Could you check a few things on this model? Use its own coordinates, in mm. Face numbers are marked on the shaded views. A direction names the side the tool comes from. Give positions to 0.01 mm unless a question says otherwise; leave off trailing zeros. Loops run counter-clockwise (first coordinate to the right, second up) from the corner with the lowest first, then second, coordinate; pieces in that order, holes last.
1. Imagine slicing it at C-C (x = 15). List the corners of the cut face in (y, z) for me, plus the area to 3 significant figures.
2. For P1, Ø6.5, axis at x = 19.5, y = 15, coming from the +Z side; P2, Ø10, axis at x = 22, z = 13.5, coming from the -Y side; P3, Ø7.5, axis at y = 8.5, z = 13.5, coming from the +X side; P4, Ø10, axis at x = 18, y = 4.5, coming from the -Z side, each with a flat end and sliding along its axis, tell me the tip position at first contact or that it passes through.
3. For the marked faces 1, 2 and 3, which set-ups out of +Z, -Z, +X, -X, +Y, -Y let a thin tool reach every point of the face, with its end or its side?
4. Thinking about a two-plate mould opening in X: for the marked faces 4, 5 and 6, which applies, +X half, -X half, draft (parallel to the pull), parting line (faces both ways), or undercut?
5. Imagine slicing it at B-B (y = 21). List the corners of the cut face in (x, z) for me (3 decimals).
6. Imagine slicing it at A-A (z = 8). List the corners of the cut face in (x, y) for me.
7. I need wall thicknesses on line 1 along X through (y, z) = (22.75, 5.75) (3 decimals); line 2 along Z through (x, y) = (25.4, 14.5) (3 decimals); line 3 along X through (y, z) = (23.75, 14.75). Which ranges of each line are inside material? Lowest first, please.
8. Imagine slicing it at D-D (z = 21.25). List the corners of the cut face in (x, y) for me.
```python
from build123d import *

# Parameters (mm, degrees)
F0_W     = 25.4
F0_H     = 25.4
F1_DEPTH = 12.7
F2_W     = 12.7
F2_H     = 12.7
F3_DEPTH = 12.7
F4_R     = 9.525
F5_DEPTH = 25.4
F6_R     = 6.35
F7_DEPTH = 25.4


with BuildPart() as f1:
    # F0 (on Right) → F1 (new body)
    with BuildSketch(Plane.YZ):
        with Locations((12.7, 12.7)):
            Rectangle(F0_W, F0_H)
    extrude(amount=F1_DEPTH)

    # F2 (on face) → F3 (join)
    with BuildSketch(Plane.YZ.offset(12.7)):
        with Locations((12.7, 12.7)):
            Rectangle(F2_W, F2_H)
    extrude(amount=F3_DEPTH)

    # F4 (on Front) → F5 (join)
    with BuildSketch(Plane.XZ):
        with Locations((25.4, 9.525)):
            Circle(F4_R)
    extrude(amount=-F5_DEPTH)

    # F6 (on face) → F7 (cut)
    with BuildSketch(Plane.XZ):
        with Locations((25.4, 9.525)):
            Circle(F6_R)
    extrude(amount=-F7_DEPTH, mode=Mode.SUBTRACT)


solid = f1.part
```
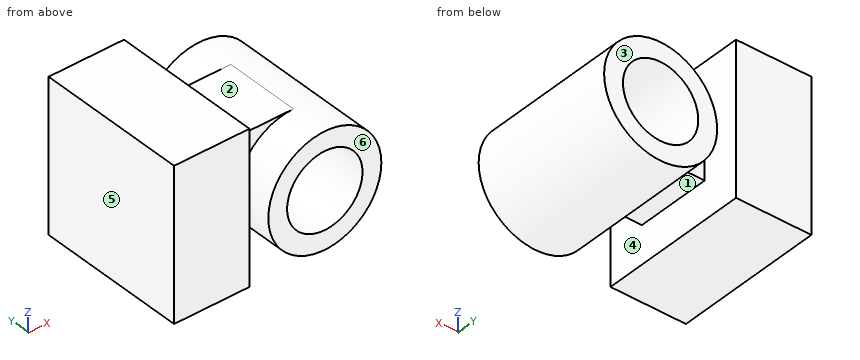
Derived:
1. outline: (6.35, 6.35) - (19.05, 6.35) - (19.05, 19.05) - (6.35, 19.05) - close
1. area: 161 mm2
2. P1: stops at z = 19.05
2. P2: stops at y = 0
2. P3: stops at x = 34.92
2. P4: stops at z = 0.31
3. face 1: -Z, +Y, -Y
3. face 2: +Z, +X, +Y, -Y
3. face 3: +Z, -Z, +X, -X, +Y
4. face 4: undercut
4. face 5: -X half
4. face 6: draft
5. outline: (0, 0) - (12.7, 0) - (12.7, 25.4) - (0, 25.4) - close; circle Ø19.05 at (25.4, 9.525); hole circle Ø12.7 at (25.4, 9.525)
6. outline: (0, 0) - (12.7, 0) - (12.7, 6.35) - (16, 6.35) - (16, 0) - (19.24, 0) - (19.24, 25.4) - (16, 25.4) - (16, 19.05) - (12.7, 19.05) - (12.7, 25.4) - (0, 25.4) - close; (31.56, 0) - (34.8, 0) - (34.8, 25.4) - (31.56, 25.4) - close
7. line 1: x = 0 to 12.7, 16.655 to 20.294, 30.506 to 34.145
7. line 2: z = 0 to 3.175, 15.875 to 19.05
7. line 3: x = 0 to 12.7, 17.44 to 21.79, 29.01 to 33.36
8. outline: (0, 0) - (12.7, 0) - (12.7, 25.4) - (0, 25.4) - close
